Geometry check sheet. Reference: drawing and pictorial views, mm from the part's lowest x, y, z. A direction names the side the tool comes from. Give positions to 0.01 mm unless a question says otherwise; leave off trailing zeros. Order: outer loops, then holes, each group sorted by start corner. A loop starts at its lowest first (then second) coordinate and runs counter-clockwise, first axis right, second up.
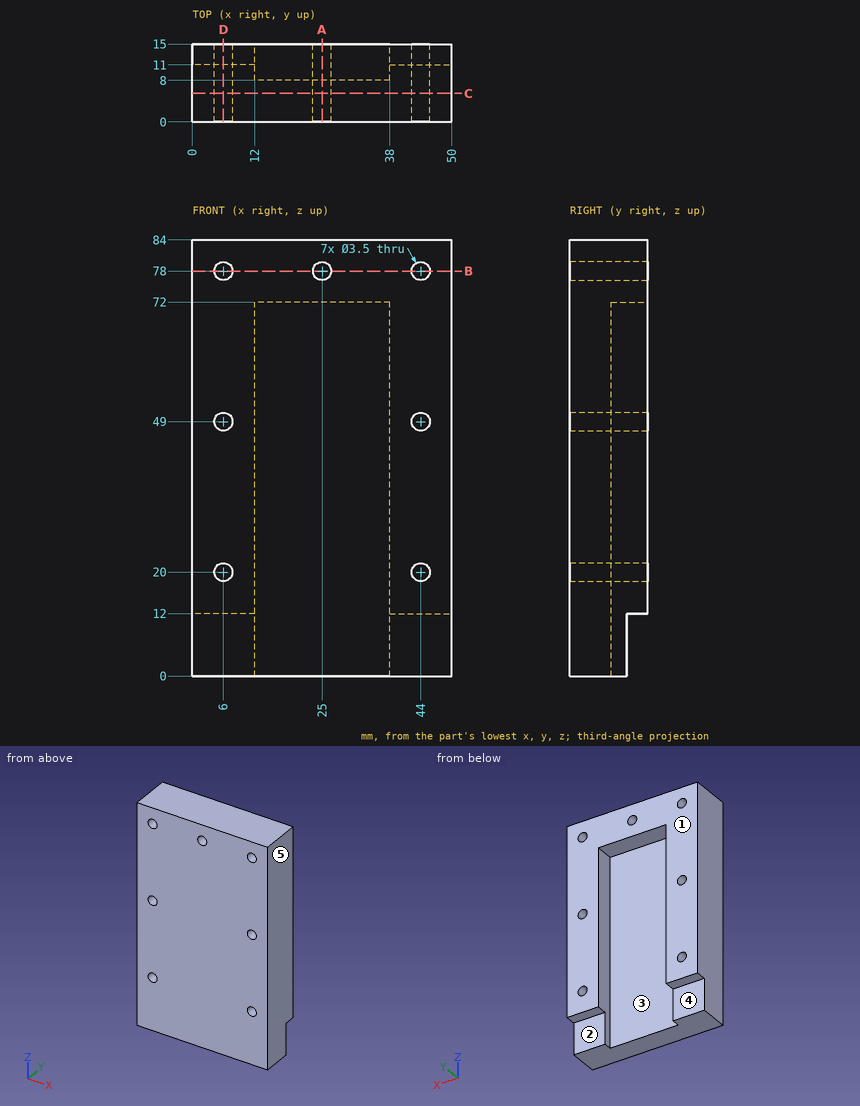
1) Section check A-A, the plane x = 25. Record the cut outline in (y, z), then the cut area to 4 significant figures.
Recorded:
outline: (0, 0) - (8, 0) - (8, 72) - (15, 72) - (15, 76.25) - (0, 76.25) - close; (0, 79.75) - (15, 79.75) - (15, 84) - (0, 84) - close
area: 703.5 mm2
2) Set-up check for the marked faces 1 and 2: record each of +Z, -Z, +X, -X, +Y, -Y from which the full face is reachable in a straight line by a thin tool's end or side.
Recorded:
face 1: +Z, -Z, +X, -X, +Y
face 2: -Z, +X, -X, +Y
3) Draft check along X on the marked faces 3, 4 and 5. Enter one of: +X half, -X half, draft (parallel to the pull), parting line (faces both ways), or undercut.
Recorded:
face 3: undercut
face 4: draft
face 5: +X half
4) Section check B-B, the plane z = 78. Record the cut outline in (x, y), then the cut area to 4 significant figures.
Recorded:
outline: (0, 0) - (4.25, 0) - (4.25, 15) - (0, 15) - close; (7.75, 0) - (23.25, 0) - (23.25, 15) - (7.75, 15) - close; (26.75, 0) - (42.25, 0) - (42.25, 15) - (26.75, 15) - close; (45.75, 0) - (50, 0) - (50, 15) - (45.75, 15) - close
area: 592.5 mm2
5) Material ranges on L1, parallel to X at y = 11.75, z = 20; L2, parallel to X at y = 3.25, z = 20; L3, parallel to X at y = 10.25, z = 78, recorded low to high.
Recorded:
L1: x = 0 to 4.25, 7.75 to 12, 38 to 42.25, 45.75 to 50
L2: x = 0 to 4.25, 7.75 to 42.25, 45.75 to 50
L3: x = 0 to 4.25, 7.75 to 23.25, 26.75 to 42.25, 45.75 to 50
6) Section check C-C, the plane y = 5.5. Record the cut outline in (x, z), then the cut area to 3 significant figures.
Recorded:
outline: (0, 0) - (50, 0) - (50, 84) - (0, 84) - close; hole circle Ø3.5 at (6, 20); hole circle Ø3.5 at (6, 49); hole circle Ø3.5 at (6, 78); hole circle Ø3.5 at (25, 78); hole circle Ø3.5 at (44, 20); hole circle Ø3.5 at (44, 49); hole circle Ø3.5 at (44, 78)
area: 4,130 mm2
7) Depth check by flat-ended pin: pin 1 Ø13 at (x, z) = (41.5, 8.5) entering from +Y; pin 2 Ø4 at (x, z) = (24, 37) entering from +Y; pin 3 Ø2 at (x, z) = (6, 49) entering from -Y; pin 4 Ø3.5 at (x, y) = (21.5, 11) entering from -Z. Enter the tip coordinate at first touch or a pass-through.
Recorded:
pin 1: stops at y = 15
pin 2: stops at y = 8
pin 3: passes through
pin 4: stops at z = 72
8) Section check D-D, the plane x = 6. Record the cut outline in (y, z), then the cut area to 3 significant figures.
Recorded:
outline: (0, 0) - (11, 0) - (11, 12) - (15, 12) - (15, 18.25) - (0, 18.25) - close; (0, 21.75) - (15, 21.75) - (15, 47.25) - (0, 47.25) - close; (0, 50.75) - (15, 50.75) - (15, 76.25) - (0, 76.25) - close; (0, 79.75) - (15, 79.75) - (15, 84) - (0, 84) - close
area: 1,050 mm2
